from build123d import *

# Parameters (mm, degrees)
SKETCH_1_W          = 120
SKETCH_1_H          = 80
EXTRUDE_1_DEPTH     = 38
SKETCH_3_W          = 117.6
SKETCH_3_H          = 77.6
CUT_EXTRUDE_1_DEPTH = 36
SKETCH_4_W          = 25.152970524
SKETCH_4_H          = 18.492901276
CUT_EXTRUDE_2_DEPTH = 10
SKETCH_7_W          = 17.413678367
SKETCH_7_H          = 5.076618726
SKETCH_7_H_2        = 5.541721388
EXTRUDE_2_DEPTH     = 0.1
SKETCH_9_W          = 27.882777132
SKETCH_9_H          = 24.878568111
CUT_EXTRUDE_4_DEPTH = 12
SKETCH_12_R         = 1.085209003
SKETCH_12_R_2       = 1.1
SKETCH_12_W         = 5.025
SKETCH_12_H         = 2.2
CUT_EXTRUDE_5_DEPTH = 12
SKETCH_13_R         = 1.35
CUT_EXTRUDE_6_DEPTH = 12
SKETCH_14_W         = 117.6
SKETCH_14_H         = 36
CUT_EXTRUDE_7_DEPTH = 10
EXTRUDE_3_DEPTH     = 5
SKETCH_16_W         = 120
SKETCH_16_H         = 38
EXTRUDE_4_DEPTH     = 2
SKETCH_17_W         = 36
SKETCH_17_H         = 83.8
EXTRUDE_5_DEPTH     = 1
EXTRUDE_6_DEPTH     = 1
SKETCH_19_W         = 120
SKETCH_19_H         = 38
EXTRUDE_7_DEPTH     = 1
EXTRUDE_START       = 2
SKETCH_20_R         = 2
SKETCH_20_R_2       = 1.085209003
SKETCH_20_R_3       = 2.001649737
SKETCH_20_R_4       = 1.1
SKETCH_20_W         = 7.2
SKETCH_20_H         = 4.2
SKETCH_20_W_2       = 5.025
SKETCH_20_H_2       = 2.2
EXTRUDE_8_DEPTH     = 2
SKETCH_22_W         = 120
SKETCH_22_H         = 88
CUT_EXTRUDE_8_DEPTH = 35


with BuildPart() as part:
    # 草图1 → 凸台-拉伸1 (new body)
    with BuildSketch(Plane.XY):
        with Locations((-463.106796117, 303.186737633)):
            Rectangle(SKETCH_1_W, SKETCH_1_H)
    extrude(amount=EXTRUDE_1_DEPTH)

    # 草图3 → 切除-拉伸1 (cut)
    with BuildSketch(Plane.XY.offset(38)):
        with Locations((-463.106796117, 303.186737633)):
            Rectangle(SKETCH_3_W, SKETCH_3_H)
    extrude(amount=-CUT_EXTRUDE_1_DEPTH, mode=Mode.SUBTRACT)

    # 草图4 → 切除-拉伸2 (cut)
    with BuildSketch(Plane(origin=(0, 0, 0), x_dir=(-1, 0, 0), z_dir=(0, 0, -1))):
        with Locations((411.924701676, 291.841861287)):
            Rectangle(SKETCH_4_W, SKETCH_4_H)
    extrude(amount=-CUT_EXTRUDE_2_DEPTH, mode=Mode.SUBTRACT)

    # 草图7 → 凸台-拉伸2 (add)
    with BuildSketch(Plane(origin=(0, 0, 0), x_dir=(-1, 0, 0), z_dir=(0, 0, -1))):
        with Locations((474.461956934, 316.64842827)):
            Rectangle(SKETCH_7_W, SKETCH_7_H)
        with Locations((474.461956934, 296.957598327)):
            Rectangle(SKETCH_7_W, SKETCH_7_H_2)
    extrude(amount=EXTRUDE_2_DEPTH)

    # 草图9 → 切除-拉伸4 (cut)
    with BuildSketch(Plane(origin=(0, 0, 0), x_dir=(-1, 0, 0), z_dir=(0, 0, -1))):
        with Locations((451.813729184, 306.747453577)):
            Rectangle(SKETCH_9_W, SKETCH_9_H)
    extrude(amount=-CUT_EXTRUDE_4_DEPTH, mode=Mode.SUBTRACT)

    # 草图12 → 切除-拉伸5 (cut)
    with BuildSketch(Plane(origin=(0, 0, -0.1), x_dir=(-1, 0, 0), z_dir=(0, 0, -1))):
        with Locations((481.368796117, 317.386737633)):
            Circle(SKETCH_12_R)
        with Locations((481.368796117, 296.186737633)):
            Circle(SKETCH_12_R_2)
        with Locations((470.281296117, 317.386737633)):
            Rectangle(SKETCH_12_W, SKETCH_12_H)
        with Locations((470.281296117, 296.186737633)):
            Rectangle(SKETCH_12_W, SKETCH_12_H)
    extrude(amount=-CUT_EXTRUDE_5_DEPTH, mode=Mode.SUBTRACT)

    # 草图13 → 切除-拉伸6 (cut)
    with BuildSketch(Plane.XY.offset(2)):
        with Locations((-475.806796117, 316.886737633)):
            Circle(SKETCH_13_R)
        with Locations((-417.806796117, 316.886737633)):
            Circle(SKETCH_13_R)
        with Locations((-417.806796117, 267.886737633)):
            Circle(SKETCH_13_R)
        with Locations((-475.806796117, 267.886737633)):
            Circle(SKETCH_13_R)
    extrude(amount=-CUT_EXTRUDE_6_DEPTH, mode=Mode.SUBTRACT)

    # 草图14 → 切除-拉伸7 (cut)
    with BuildSketch(Plane.XZ.offset(-341.986737633)):
        with Locations((-463.106796117, 20)):
            Rectangle(SKETCH_14_W, SKETCH_14_H)
    extrude(amount=-CUT_EXTRUDE_7_DEPTH, mode=Mode.SUBTRACT)

    # 草图15 → 凸台-拉伸3 (add)
    with BuildSketch(Plane(origin=(0, 343.186737633, 0), x_dir=(1, 0, 0), z_dir=(0, 1, 0))):
        Polygon((-521.906796117, -2), (-404.306796117, -2), (-404.306796117, -38), (-403.106796117, -38), (-403.106796117, 0), (-523.106796117, 0), (-523.106796117, -38), (-521.906796117, -38), align=None)
    extrude(amount=EXTRUDE_3_DEPTH)

    # 草图16 → 凸台-拉伸4 (add)
    with BuildSketch(Plane(origin=(0, 348.186737633, 0), x_dir=(1, 0, 0), z_dir=(0, 1, 0))):
        with Locations((-463.106796117, -19)):
            Rectangle(SKETCH_16_W, SKETCH_16_H)
    extrude(amount=EXTRUDE_4_DEPTH)

    # 草图17 → 凸台-拉伸5 (add)
    with BuildSketch(Plane(origin=(-521.906796117, 0, 0), x_dir=(0, 0, -1), z_dir=(1, 0, 0))):
        with Locations((-20, 306.286737633)):
            Rectangle(SKETCH_17_W, SKETCH_17_H)
    extrude(amount=EXTRUDE_5_DEPTH)

    # 草图18 → 凸台-拉伸6 (add)
    with BuildSketch(Plane.ZY.offset(404.306796117)):
        Polygon((10, 301.088311925), (10, 282.595410649), (2, 282.595410649), (2, 264.386737633), (38, 264.386737633), (38, 348.186737633), (2, 348.186737633), (2, 301.088311925), align=None)
    extrude(amount=EXTRUDE_6_DEPTH)

    # 草图19 → 凸台-拉伸7 (add)
    with BuildSketch(Plane.XZ.offset(-263.186737633)):
        with Locations((-463.106796117, 19)):
            Rectangle(SKETCH_19_W, SKETCH_19_H)
    extrude(amount=EXTRUDE_7_DEPTH)

    # 草图20 → 凸台-拉伸8 (add)
    # profile 1 of 4: a face of its own
    with BuildSketch(Plane(origin=(0, 0, -0.1), x_dir=(-1, 0, 0), z_dir=(0, 0, -1)).offset(EXTRUDE_START)):
        with Locations(Location((481.368796117, 317.386737633, 0), (0, 0, 115.841932763))):
            Circle(SKETCH_20_R)
        with Locations((481.368796117, 317.386737633)):
            Circle(SKETCH_20_R_2, mode=Mode.SUBTRACT)
    # profile 2 of 4: a face of its own
    with BuildSketch(Plane(origin=(0, 0, -0.1), x_dir=(-1, 0, 0), z_dir=(0, 0, -1)).offset(EXTRUDE_START)):
        with Locations(Location((481.368796117, 296.186737633, 0), (0, 0, 267.673619076))):
            Circle(SKETCH_20_R_3)
        with Locations((481.368796117, 296.186737633)):
            Circle(SKETCH_20_R_4, mode=Mode.SUBTRACT)
    # profile 3 of 4: a face of its own
    with BuildSketch(Plane(origin=(0, 0, -0.1), x_dir=(-1, 0, 0), z_dir=(0, 0, -1)).offset(EXTRUDE_START)):
        with Locations((470.395177276, 317.386737633)):
            Rectangle(SKETCH_20_W, SKETCH_20_H)
        with Locations((470.281296117, 317.386737633)):
            Rectangle(SKETCH_20_W_2, SKETCH_20_H_2, mode=Mode.SUBTRACT)
    # profile 4 of 4: a face of its own
    with BuildSketch(Plane(origin=(0, 0, -0.1), x_dir=(-1, 0, 0), z_dir=(0, 0, -1)).offset(EXTRUDE_START)):
        with Locations((470.325427447, 296.233937818)):
            Rectangle(SKETCH_20_W, SKETCH_20_H)
        with Locations((470.281296117, 296.186737633)):
            Rectangle(SKETCH_20_W_2, SKETCH_20_H_2, mode=Mode.SUBTRACT)
    extrude(amount=-EXTRUDE_8_DEPTH)

    # 草图22 → 切除-拉伸8 (cut)
    with BuildSketch(Plane.XY.offset(38)):
        with Locations((-463.106796117, 306.186737633)):
            Rectangle(SKETCH_22_W, SKETCH_22_H)
    extrude(amount=-CUT_EXTRUDE_8_DEPTH, mode=Mode.SUBTRACT)


solid = part.part
Verification items for the finished model (mm, model axes). A direction names the side the tool comes from. Round coordinates to 2 decimals unless told otherwise and drop trailing zeros. Loops run counter-clockwise (first coordinate to the right, second up) from the corner with the lowest first, then second, coordinate; pieces in that order, holes last. Notation, with made-up numbers: (75, 5) - (85, 5) arc R23 cw to (85, 42) - close; hole circle Ø8 at (33.5, 8.25). An arc over 180 degrees is marked (long way). Answer in a Markdown table with one row per item. Add a question column.
Q1. Section check A-A on x = -440. Enter the section's corners in (y, z).
Q2. Release check for a two-part mould opening along X. For faces 1 (the face through (-481.892, 294.255, -1.114)), 2 (the face through (-403.107, 273, 1)), 3 (the face through (-521.2, 306.4, 3)), 4 (the face through (-419.155, 267.946, 1.014)) record: pulls with the +X half, pulls with the -X half, needs draft (parallel to the pull), parting line crosses it, or undercut.
Q3. Material ranges on line 1 (Y direction, x = -468.5, z = -0.65); line 2 (Y direction, x = -481.5, z = -1.75); line 3 (Y direction, x = -444, z = 0.4), recorded low to high.
Q4. Gauge pin test, flat ends, axial feed: pin 1 (2 mm diameter, centred on y = 318, z = -1.5, fed in from +X); pin 2 (12 mm diameter, centred on x = -445.5, y = 286, fed in from -Z); pin 3 (3 mm diameter, centred on x = -475.81, y = 316.89, fed in from +Z). Record the tip position at first contact, or that the pin passes through.
Q5. Section check B-B on y = 302.5. Enter the section's corners in (x, z), plus the area to 3 significant figures.
Q6. Tool access check on faces 5 (the face through (-470, 318.487, 0)), 6 (the face through (-482.16, 315.55, -1.11)), 7 (the face through (-414, 301.088, 1)), 8 (the face through (-477, 306, 2)). Record the directions out of +Z, -Z, +X, -X, +Y, -Y that give a thin tool (end or side, any length) a straight path to the whole face; none if there is none.
Q7. Section check C-C on x = -499.5. Enter the section's corners in (y, z), plus the area to 3 significant figures.
Q8. Section check D-D on z = 0.85. State how many separate pieces and enclosed holes the cut face has, plus the area to 3 significant figures.
Found:
| question | item | result |
|---|---|---|
| 1 | outline | (262.19, 0) - (294.31, 0) - (294.31, 2) - (264.39, 2) - (264.39, 3) - (262.19, 3) - close; (319.19, 0) - (350.19, 0) - (350.19, 3) - (348.19, 3) - (348.19, 2) - (319.19, 2) - close |
| 2 | face 1 | undercut |
| 2 | face 2 | pulls with the +X half |
| 2 | face 3 | needs draft |
| 2 | face 4 | undercut |
| 3 | line 1 | y = 294.13 to 295.09, 297.29 to 298.33, 315.29 to 316.29, 318.49 to 319.49 |
| 3 | line 2 | y = 294.19 to 295.09, 297.28 to 298.18, 315.39 to 316.31, 318.46 to 319.38 |
| 3 | line 3 | y = 262.19 to 294.31, 319.19 to 350.19 |
| 4 | pin 1 | stops at x = -466.8 |
| 4 | pin 2 | stops at z = 0 |
| 4 | pin 3 | stops at z = 2 |
| 5 | outline | (-523.11, 0) - (-465.76, 0) - (-465.76, 2) - (-520.91, 2) - (-520.91, 3) - (-523.11, 3) - close; (-437.87, 0) - (-403.11, 0) - (-403.11, 3) - (-405.31, 3) - (-405.31, 2) - (-437.87, 2) - close |
| 5 | area | 189 mm² |
| 6 | face 5 | +Z, -Z |
| 6 | face 6 | -Z |
| 6 | face 7 | +Z, -Z, +X |
| 6 | face 8 | +Z |
| 7 | outline | (262.19, 0) - (350.19, 0) - (350.19, 3) - (348.19, 3) - (348.19, 2) - (264.39, 2) - (264.39, 3) - (262.19, 3) - close |
| 7 | area | 180 mm² |
| 8 | separate pieces | 1 |
| 8 | enclosed holes | 9 |
| 8 | area | 9,420 mm² |
